For this review, take the finished solid that the model builds, in its own axes (mm). Round coordinates to 2 decimals unless told otherwise and drop trailing zeros. Order: outer loops, then holes, each group sorted by start corner. A loop starts at its lowest first (then second) coordinate and runs counter-clockwise, first axis right, second up. Notation, with made-up numbers: M 59,35 L 110,35 A34 ccw 110,71 Z; hole C -7.5,50 d10. An arc over 180 degrees is marked long. Put each result on its own line as item: value.
from build123d import *

# Parameters (mm, degrees)
SKETCH1_R           = 76.2
SKETCH1_R_2         = 19.05
BOSS_EXTRUDE1_DEPTH = 12.7
CIRPATTERN1_COUNT   = 2
FILLET1_R           = 101.6
CUT_EXTRUDE2_DEPTH  = 13.7
FILLET2_R           = 6.35


with BuildPart() as part:
    # Sketch1 → Boss-Extrude1 (new body)
    with BuildSketch(Plane(origin=(0, 0, 0), x_dir=(1, 0, 0), z_dir=(0, 1, 0))):
        with BuildLine():
            ThreePointArc((-461.937950379, 266.7), (-515.224835743, 138.054078658), (-533.4, 0))
            Line((-533.4, 0), (-431.8, 27.223637951))
            ThreePointArc((-431.8, 27.223637951), (-391.951998133, 36.135119544), (-351.499222019, 41.689456733))
            Line((-351.499222019, 41.689456733), (-14.198340678, 73.716868009))
            ThreePointArc((-14.198340678, 73.716868009), (-73.012974959, 93.516111014), (-97.595715318, 150.497336919))
            Line((-97.595715318, 150.497336919), (-323.429158368, 129.053987789))
            ThreePointArc((-323.429158368, 129.053987789), (-424.955630689, 165.402632783), (-461.937950379, 266.7))
        make_face()
        with Locations((-21.401289496, 149.575667949)):
            Circle(SKETCH1_R)
        with Locations((-21.401289496, 149.575667949)):
            Circle(SKETCH1_R_2, mode=Mode.SUBTRACT)
    boss_extrude1 = extrude(amount=BOSS_EXTRUDE1_DEPTH)

    # CirPattern1: Boss-Extrude1 ×2 about axis
    cirpattern1_axis = Axis((-21.401289496, 0, -149.575667949), (0, 1, 0))
    for i in range(1, CIRPATTERN1_COUNT):
        add(boss_extrude1.rotate(cirpattern1_axis, i * 360 / CIRPATTERN1_COUNT))

    # Fillet1
    fillet1_edges = [part.edges().sort_by_distance(p)[0] for p in [
        (-97.595715318, 6.35, -150.497336919),
        (54.793136326, 6.35, -148.653998979),
    ]]
    fillet(fillet1_edges, radius=FILLET1_R)

    # Sketch3 → Cut-Extrude2 (cut, through all)
    with BuildSketch(Plane(origin=(0, 12.7, 0), x_dir=(1, 0, 0), z_dir=(0, 1, 0))):
        with BuildLine():
            ThreePointArc((-354.80057356, 76.458073372), (-356.713011165, 85.800166676), (-358.363729661, 95.192038339))
            ThreePointArc((-358.363729661, 95.192038339), (-421.769213749, 118.496456117), (-470.148687166, 165.642801175))
            ThreePointArc((-470.148687166, 165.642801175), (-486.927538331, 106.671917768), (-496.339895031, 46.087245799))
            Line((-496.339895031, 46.087245799), (-440.83925515, 60.958597434))
            ThreePointArc((-440.83925515, 60.958597434), (-398.143908594, 70.506850222), (-354.80057356, 76.458073372))
        make_face()
        with BuildLine():
            ThreePointArc((398.036676158, 238.192738464), (355.341329602, 228.644485675), (311.997994568, 222.693262526))
            ThreePointArc((311.997994568, 222.693262526), (313.910432173, 213.351169222), (315.561150668, 203.959297559))
            ThreePointArc((315.561150668, 203.959297559), (378.966634757, 180.654879781), (427.346108174, 133.508534723))
            ThreePointArc((427.346108174, 133.508534723), (444.124959338, 192.47941813), (453.537316039, 253.064090099))
            Line((453.537316039, 253.064090099), (398.036676158, 238.192738464))
        make_face()
    extrude(amount=-CUT_EXTRUDE2_DEPTH, mode=Mode.SUBTRACT)

    # Fillet2
    fillet2_edges = [part.edges().sort_by_distance(p)[0] for p in [
        (-354.80057356, 6.35, -76.458073372),
        (-496.339895031, 6.35, -46.087245799),
        (-470.148687166, 6.35, -165.642801175),
        (-358.363729661, 6.35, -95.192038339),
        (311.997994568, 6.35, -222.693262526),
        (453.537316039, 6.35, -253.064090099),
        (427.346108174, 6.35, -133.508534723),
        (315.561150668, 6.35, -203.959297559),
    ]]
    fillet(fillet2_edges, radius=FILLET2_R)


solid = part.part
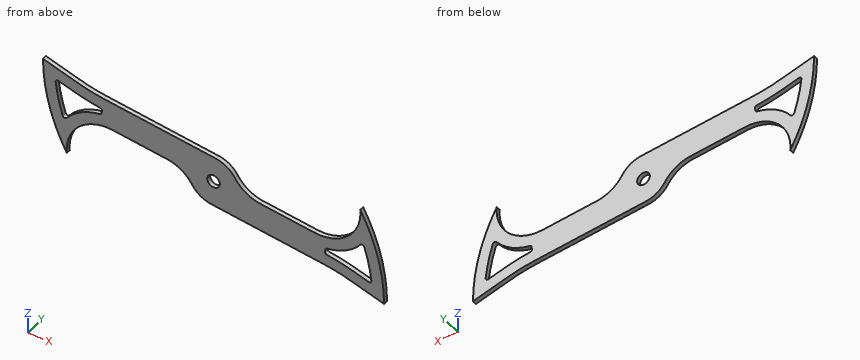
(1) Add section B-B on y = 4.75. State how many separate pieces and enclosed holes the cut face has, then the cut area to 3 significant figures.
A:
separate pieces: 1
enclosed holes: 3
area: 102,000 mm2
(2) Insertion check: pin 1 Ø4 at (y, z) = (3.5, -61.5) entering from -X; pin 2 Ø1.5 at (y, z) = (5.5, -115) entering from -X; pin 3 Ø4 at (x, y) = (76.5, 7) entering from +Z. Each pin has a flat end and moves straight along its axis. Give the tip position at first contact, or say it passes through.
A:
pin 1: stops at x = -530.07
pin 2: stops at x = -521.02
pin 3: stops at z = -139.79
(3) Add section C-C on x = -397. Give the boundary of the cut face in (y, z).
A:
outline: M 0,-144.41 L 12.7,-144.41 L 12.7,-105.72 L 0,-105.72 Z; M 0,-70.71 L 12.7,-70.71 L 12.7,-35.2 L 0,-35.2 Z
(4) Add section A-A on x = 351.5. Give the boundary of the cut face in (y, z), then the cut area to 3 significant figures.
A:
outline: M 0,-263.45 L 12.7,-263.45 L 12.7,-227.97 L 0,-227.97 Z; M 0,-194.51 L 12.7,-194.51 L 12.7,-156.2 L 0,-156.2 Z
area: 937 mm2
(5) Add section D-D on x = 99. Give the boundary of the cut face in (y, z).
A:
outline: M 0,-237.55 L 12.7,-237.55 L 12.7,-150.87 L 0,-150.87 Z
(6) To check wall thickness, follow L1, parallel to X at y = 8.25, z = -208.5; L2, parallel to X at y = 5, z = -193; L3, parallel to Z at x = 395.5, y = 4.25. State the ranges of each line that lie inside material, in increasing order.
A:
L1: x = -490.96 to -453.42, -69.72 to 314.8, 447.36 to 482.84
L2: x = -497.26 to -446, -84.02 to 355.23, 444.24 to 479.93
L3: z = -273.67 to -237.52, -168.72 to -118.14
